Autodesk Inventor part; units mm, degrees
ref_plane "YZ Plane" through (0, 0, 0) normal (1, 0, 0) x (0, 1, 0)
ref_plane "XZ Plane" through (0, 0, 0) normal (0, 1, 0) x (-1, 0, 0)
ref_plane "XY Plane" through (0, 0, 0) normal (0, 0, 1) x (1, 0, 0)
sketch "Sketch1" plane through (0, 0, 0) normal (0, 1, 0) x (-1, 0, 0)
  circle A0 centre (0, 0) radius 6.15
  line L0 (10, 13) -> (-10, 13)
  line L1 (-10, 13) -> (-10, -13)
  line L2 (-10, -13) -> (10, -13)
  line L3 (10, -13) -> (10, 13)
  dimension "d0" = 12.3
  dimension "d1" = 10
  dimension "d2" = 10
  dimension "d3" = 13
  dimension "d4" = 13
extrude "Extrusion1" add sketch "Sketch1" along normal blind 66
sketch "Sketch2" plane through (10, 0, 13) normal (1, 0, 0) x (0, 0, -1)
  circle A0 centre (13, 5) radius 1.45
  line L0 (0, 0) -> (26, 0)
  circle A1 centre (13, 60) radius 1.45
  line L1 (0, 0) -> (0, 66)
  point P0 (13, 0)
  dimension "d7" = 2.9
  dimension "d8" = 5
  dimension "d9" = 2.9
  dimension "d11" = 13
  dimension "d12" = 13
  dimension "d41" = 55
extrude "Extrusion2" cut sketch "Sketch2" against normal blind 55
sketch "Sketch3" plane through (10, 0, 13) normal (1, 0, 0) x (0, 0, -1)
  circle A0 centre (13, 5) radius 1.45
  circle A1 centre (13, 60) radius 1.45
  line L0 (0, 0) -> (26, 0)
  line L1 (26, 0) -> (26, 66)
  line L2 (0, 66) -> (26, 66)
  line L3 (0, 0) -> (0, 66)
  circle A2 centre (13, 60) radius 5.45
  circle A3 centre (13, 5) radius 5.45
  circle A4 centre (4, 46) radius 1.6
  circle A5 centre (22, 46) radius 1.6
  circle A6 centre (4, 4) radius 1.6
  circle A7 centre (22, 4) radius 1.6
  point P0 (13, 0)
  dimension "d15" = 4
  dimension "d16" = 4
  dimension "d19" = 3.2
  dimension "d20" = 3.2
  dimension "d21" = 3.2
  dimension "d22" = 3.2
  dimension "d23" = 4
  dimension "d24" = 4
  dimension "d25" = 4
  dimension "d26" = 4
extrude "Extrusion3" add sketch "Sketch3" along normal blind 15 contours A3 L0 | L0 A3 | A2
sketch "Sketch6" plane through (-10, 0, 13) normal (0, 0, 1) x (1, 0, 0)
  line L0 (20, 66) -> (0, 66)
  line L1 (20, 0) -> (0, 0)
  line L2 (0, 66) -> (5, 66)
  line L3 (5, 66) -> (5, 0)
  line L4 (5, 0) -> (0, 0)
  line L5 (0, 0) -> (0, 66)
  point P0 (10, 0)
  dimension "d31" = 5
extrude "Extrusion6" add sketch "Sketch6" along normal blind 5
sketch "Sketch7" plane through (10, 0, -13) normal (0, 0, -1) x (-1, 0, 0)
  line L0 (20, 66) -> (20, 0)
  line L1 (20, 0) -> (15, 0)
  line L2 (20, 66) -> (15, 66)
  line L3 (15, 66) -> (15, 0)
  line L4 (15, 0) -> (20, 0)
  line L5 (20, 0) -> (20, 66)
  point P0 (10, 0)
  dimension "d34" = 5
extrude "Extrusion7" add sketch "Sketch7" along normal blind 5
sketch "Sketch8" plane through (0, 0, 0) normal (0, -1, 0) x (1, 0, 0)
  line L0 (10, 13) -> (10, -13)
  line L1 (-10, 18) -> (-10, -18)
  line L2 (10, 13) -> (-10, 13)
  line L3 (-10, 13) -> (-10, 3)
  line L4 (-10, 3) -> (10, 3)
  line L5 (10, 3) -> (10, 13)
  line L6 (10, -13) -> (-5, -13)
  line L7 (10, -13) -> (-10, -13)
  line L8 (-10, -13) -> (-10, -3)
  line L9 (-10, -3) -> (10, -3)
  line L10 (10, -3) -> (10, -13)
  point P0 (0, 0)
  point P1 (10, -3)
  point P2 (-10, -3)
  dimension "d37" = 10
  dimension "d38" = 10
extrude "Extrusion8" add sketch "Sketch8" along normal blind 2 contours L0 L4 L1 L2 | L0 L6 L7 L1 L9
properties part number "Tube_outerhole_template_large_p1"
CAD build for the part. Positions are in the model's coordinates, mm. A direction names the side the tool comes from. Round coordinates to 2 decimals unless told otherwise and drop trailing zeros. Order: outer loops, then holes, each group sorted by start corner. A loop starts at its lowest first (then second) coordinate and runs counter-clockwise, first axis right, second up. Notation, with made-up numbers: (-36.5, 5.5) -> (-24.5, 5.5) arc R21 cw to (-24.5, 24.5) -> close; hole circle Ø9 at (20.5, -34). An arc over 180 degrees is marked (long way). Write item = value, one per line.
(1) Flat gauge pins, fed straight in: P1, Ø2.5, axis at x = -7.5, z = -1, coming from the -Y side; P2, Ø2.5, axis at y = 46.5, z = -16.5, coming from the +X side; P3, Ø0.6, axis at x = 3.5, y = -1.5, coming from the +Z side. Where does each tip first touch, or does it go through?
Answers follow:
P1 = 0
P2 = -5
P3 = 13
(2) Drill centre lines: L1, parallel to Y at x = -8.15, z = 0; L2, parallel to X at y = 29, z = 0; L3, parallel to Z at x = 19.75, y = 5. Where is each one in solid material? Low to high.
Answers follow:
L1 = 0 to 3.55, 6.45 to 58.55, 61.45 to 66
L2 = -10 to -6.15, 6.15 to 10
L3 = -5.45 to -1.45, 1.45 to 5.45
(3) Cut at B-B (y = 60). Write the cut outline in (x, z), plus the area to 3 significant figures.
Answers follow:
outline = (-10, -18) -> (-5, -18) -> (-5, -13) -> (10, -13) -> (10, -5.45) -> (25, -5.45) -> (25, -1.45) -> (5.98, -1.45) arc R6.15 cw to (-5.98, -1.45) -> (-10, -1.45) -> close; (-10, 1.45) -> (-5.98, 1.45) arc R6.15 cw to (5.98, 1.45) -> (25, 1.45) -> (25, 5.45) -> (10, 5.45) -> (10, 13) -> (-5, 13) -> (-5, 18) -> (-10, 18) -> close
area = 549 mm²
(4) Cut at C-C (y = 20.5). Write the cut outline in (x, z).
Answers follow:
outline = (-10, -18) -> (-5, -18) -> (-5, -13) -> (10, -13) -> (10, 13) -> (-5, 13) -> (-5, 18) -> (-10, 18) -> close; hole circle Ø12.3 at (0, 0)
(5) Pull direction Y, two halves, no side cores. Call faces 1 (the flat face through (-8, 0, 0)), 2 (the flat face through (2, 32, 13)), 3 (the cylindrical face through (17.4, 56.3, 4)), 4 (the cylindrical face through (-7.96, 3.584, 0.314)): +Y half, -Y half, draft (parallel to the pull), parting line (faces both ways), or undercut.
Answers follow:
face_1 = -Y half
face_2 = draft
face_3 = undercut
face_4 = undercut
(6) 3-axis set-ups, long thin cutter, end or side, ignore diameter. For faces 5 (the cylindrical face through (17.395, 3.363, -5.198)), 6 (the flat face through (-8, 0, 16)), 7 (the flat face through (0, 0, 4)), 8 (the flat face through (-5, 33, -15)): which of +Z, -Z, +X, -X, +Y, -Y reach the whole face in a straight line?
Answers follow:
face_5 = +X
face_6 = +Z, +X, -X, -Y
face_7 = +Y
face_8 = -Z, +X, +Y, -Y
(7) Cut at D-D (x = 14). Write the cut outline in (y, z).
Answers follow:
outline = circle Ø10.9 at (5, 0); circle Ø10.9 at (60, 0); hole circle Ø2.9 at (5, 0); hole circle Ø2.9 at (60, 0)
(8) Cut at A-A (x = 0). Write the cut outline in (y, z).
Answers follow:
outline = (-2, -13) -> (66, -13) -> (66, -6.15) -> (0, -6.15) -> (0, -3) -> (-2, -3) -> close; (-2, 3) -> (0, 3) -> (0, 6.15) -> (66, 6.15) -> (66, 13) -> (-2, 13) -> close
